Input: part model. Units: mm. Frame: model coordinates. A direction names the side the tool comes from. Give positions to 0.01 mm unless a question says otherwise; leave off trailing zeros. Write each loop counter-clockwise with the first axis right and the second up, starting at its lowest first coordinate (ties: lowest second). Pieces come first, ordered by that corner, then holes. Notation, with made-up numbers: (-1.5, -29) - (21.5, -29) arc R19 ccw to (21.5, -22) - close; hole circle Ø7 at (88.5, 82). An arc over 180 degrees is marked (long way). Use a Markdown table: item, result. Add a question column.
1. Mould query, pull axis X, two halves, no side actions, for faces 3 (the cylindrical face through (62.6, 0.99, 62.46)), 4 (the cylindrical face through (-62.46, 0.99, 62.6)), 5 (the cylindrical face through (46.039, 0.986, 44.214)). Classes: released by +X, released by -X, zero draft, split by the parting line, or undercut.
2. Material intervals for probe 1 along X at (y, z) = (0.6, 6); probe 2 along X at (y, z) = (1.95, 8); probe 3 along X at (y, z) = (1.6, 18), sorted ascending.
3. Section query C-C, the plane z = 23.5. Return loops of the section in (x, y), plus the area to 3 significant figures.
4. Section query D-D, the plane x = -41.5. Return loops of the section in (y, z), plus the area to 3 significant figures.
5. Section query B-B, the plane x = -24. Return loops of the section in (y, z).
6. Pin query (flat end, axial travel): pin 1 (2 mm diameter, centred on x = 45.96, z = -45.96, fed in from -Y). Return the tip coordinate at first contact, or that it passes through.
7. Section query A-A, the plane z = -40. Return loops of the section in (x, y).
8. Set-up query: faces 1 (the flat face through (15, 2, -30)), 2 (the flat face through (-28.316, 0.986, -45.62)). Return all of +Z, -Z, +X, -X, +Y, -Y with unobstructed straight access to the full face (end or side cutting, diameter ignored); none if empty.
```python
from build123d import *

# Parameters (mm, degrees)
SKETCH_1_R      = 1.75
SKETCH_1_W      = 32
SKETCH_1_H      = 32
EXTRUDE_1_DEPTH = 2


with BuildPart() as part:
    # 草图1 → 凸台-拉伸1 (new body)
    with BuildSketch(Plane(origin=(0, 0, 0), x_dir=(1, 0, 0), z_dir=(0, 1, 0))):
        with BuildLine():
            Line((-56.568542495, 65), (56.568542495, 65))
            ThreePointArc((56.568542495, 65), (62.530483272, 62.530483272), (65, 56.568542495))
            Line((65, 56.568542495), (65, -56.568542495))
            ThreePointArc((65, -56.568542495), (62.530483272, -62.530483272), (56.568542495, -65))
            Line((56.568542495, -65), (-56.568542495, -65))
            ThreePointArc((-56.568542495, -65), (-62.530483272, -62.530483272), (-65, -56.568542495))
            Line((-65, -56.568542495), (-65, 56.568542495))
            ThreePointArc((-65, 56.568542495), (-62.530483272, 62.530483272), (-56.568542495, 65))
        make_face()
        with Locations(Location((-56.568542495, 56.568542495, 0), (0, 0, 270))):
            Circle(SKETCH_1_R, mode=Mode.SUBTRACT)
        with Locations(Location((56.568542495, 56.568542495, 0), (0, 0, 270))):
            Circle(SKETCH_1_R, mode=Mode.SUBTRACT)
        with Locations(Location((56.568542495, -56.568542495, 0), (0, 0, 270))):
            Circle(SKETCH_1_R, mode=Mode.SUBTRACT)
        with Locations(Location((-56.568542495, -56.568542495, 0), (0, 0, 270))):
            Circle(SKETCH_1_R, mode=Mode.SUBTRACT)
        with Locations(Location((45.961940777, 45.961940777, 0), (0, 0, 270))):
            Circle(SKETCH_1_R, mode=Mode.SUBTRACT)
        with Locations(Location((45.961940777, -45.961940777, 0), (0, 0, 270))):
            Circle(SKETCH_1_R, mode=Mode.SUBTRACT)
        with Locations(Location((-45.961940777, -45.961940777, 0), (0, 0, 270))):
            Circle(SKETCH_1_R, mode=Mode.SUBTRACT)
        with Locations(Location((-45.961940777, 45.961940777, 0), (0, 0, 270))):
            Circle(SKETCH_1_R, mode=Mode.SUBTRACT)
        with BuildLine():
            Line((-12.13091169, 33.271867745), (-44.961628787, 58.318542495))
            Line((-44.961628787, 58.318542495), (44.961628787, 58.318542495))
            Line((44.961628787, 58.318542495), (12.13091169, 33.271867745))
            ThreePointArc((12.13091169, 33.271867745), (0, 29.172841978), (-12.13091169, 33.271867745))
        make_face(mode=Mode.SUBTRACT)
        with BuildLine():
            Line((33.271867745, 12.13091169), (58.318542495, 44.961628787))
            Line((58.318542495, 44.961628787), (58.318542495, -44.961628787))
            Line((58.318542495, -44.961628787), (33.271867745, -12.13091169))
            ThreePointArc((33.271867745, -12.13091169), (29.172841978, 0), (33.271867745, 12.13091169))
        make_face(mode=Mode.SUBTRACT)
        with BuildLine():
            Line((-33.271867745, 12.13091169), (-58.318542495, 44.961628787))
            Line((-58.318542495, 44.961628787), (-58.318542495, -44.961628787))
            Line((-58.318542495, -44.961628787), (-33.271867745, -12.13091169))
            ThreePointArc((-33.271867745, -12.13091169), (-29.172841978, 0), (-33.271867745, 12.13091169))
        make_face(mode=Mode.SUBTRACT)
        with BuildLine():
            Line((12.13091169, -33.271867745), (44.961628787, -58.318542495))
            Line((44.961628787, -58.318542495), (-44.961628787, -58.318542495))
            Line((-44.961628787, -58.318542495), (-12.13091169, -33.271867745))
            ThreePointArc((-12.13091169, -33.271867745), (0, -29.172841978), (12.13091169, -33.271867745))
        make_face(mode=Mode.SUBTRACT)
        Rectangle(SKETCH_1_W, SKETCH_1_H, mode=Mode.SUBTRACT)
    extrude(amount=EXTRUDE_1_DEPTH)


solid = part.part
```
Result sheet:
| question | item | result |
|---|---|---|
| 1 | face 3 | released by +X |
| 1 | face 4 | released by -X |
| 1 | face 5 | undercut |
| 2 | probe 1 | x = -65 to -58.32, -30.09 to -16, 16 to 30.09, 58.32 to 65 |
| 2 | probe 2 | x = -65 to -58.32, -30.84 to -16, 16 to 30.84, 58.32 to 65 |
| 2 | probe 3 | x = -65 to -58.32, -37.75 to 37.75, 58.32 to 65 |
| 3 | outline | (-65, 0) - (-58.32, 0) - (-58.32, 2) - (-65, 2) - close; (-41.95, 0) - (41.95, 0) - (41.95, 2) - (-41.95, 2) - close; (58.32, 0) - (65, 0) - (65, 2) - (58.32, 2) - close |
| 3 | area | 195 mm² |
| 4 | outline | (0, -65) - (2, -65) - (2, -58.32) - (0, -58.32) - close; (0, -55.68) - (2, -55.68) - (2, -22.92) - (0, -22.92) - close; (0, 22.92) - (2, 22.92) - (2, 55.68) - (0, 55.68) - close; (0, 58.32) - (2, 58.32) - (2, 65) - (0, 65) - close |
| 4 | area | 158 mm² |
| 5 | outline | (0, -65) - (2, -65) - (2, -58.32) - (0, -58.32) - close; (0, -42.33) - (2, -42.33) - (2, 42.33) - (0, 42.33) - close; (0, 58.32) - (2, 58.32) - (2, 65) - (0, 65) - close |
| 6 | pin 1 | passes through |
| 7 | outline | (-65, 0) - (-58.32, 0) - (-58.32, 2) - (-65, 2) - close; (-54.53, 0) - (-20.95, 0) - (-20.95, 2) - (-54.53, 2) - close; (20.95, 0) - (54.53, 0) - (54.53, 2) - (20.95, 2) - close; (58.32, 0) - (65, 0) - (65, 2) - (58.32, 2) - close |
| 8 | face 1 | +Z, -Z, +X, -X, +Y |
| 8 | face 2 | +Y, -Y |
